Input: part model. Units: mm. Frame: model coordinates. A direction names the side the tool comes from. Give positions to 0.01 mm unless a question says otherwise; leave off trailing zeros. Order: outer loops, then holes, each group sorted by start corner. A loop starts at its lowest first (then second) coordinate and runs counter-clockwise, first axis right, second up.
```python
from build123d import *

# Parameters (mm, degrees)
SKETCH1_W           = 52
SKETCH1_H           = 40.7
SKETCH1_R           = 1.8
BOSS_EXTRUDE1_DEPTH = 1.6
SKETCH2_W           = 11
SKETCH2_H           = 10.7
SKETCH2_H_2         = 10
SKETCH2_H_3         = 13
BOSS_EXTRUDE2_DEPTH = 10
SKETCH3_R           = 1
CUT_EXTRUDE1_DEPTH  = 67.786899913


with BuildPart() as part:
    # Sketch1 → Boss-Extrude1 (new body)
    with BuildSketch(Plane(origin=(0, 0, 0), x_dir=(1, 0, 0), z_dir=(0, 1, 0))):
        with Locations((26, 20.35)):
            Rectangle(SKETCH1_W, SKETCH1_H)
        with Locations(Location((3.8, 36.85, 0), (0, 0, 270))):
            Circle(SKETCH1_R, mode=Mode.SUBTRACT)
        with Locations(Location((48.2, 36.85, 0), (0, 0, 270))):
            Circle(SKETCH1_R, mode=Mode.SUBTRACT)
        with Locations(Location((48.2, 3.85, 0), (0, 0, 270))):
            Circle(SKETCH1_R, mode=Mode.SUBTRACT)
        with Locations(Location((3.8, 3.85, 0), (0, 0, 270))):
            Circle(SKETCH1_R, mode=Mode.SUBTRACT)
    extrude(amount=BOSS_EXTRUDE1_DEPTH)

    # Sketch2 → Boss-Extrude2 (add)
    with BuildSketch(Plane(origin=(0, 1.6, 0), x_dir=(1, 0, 0), z_dir=(0, 1, 0))):
        with Locations((46.5, 15.35)):
            Rectangle(SKETCH2_W, SKETCH2_H)
        with Locations((5.5, 27.7)):
            Rectangle(SKETCH2_W, SKETCH2_H_2)
        with Locations((5.5, 14.2)):
            Rectangle(SKETCH2_W, SKETCH2_H_3)
    extrude(amount=BOSS_EXTRUDE2_DEPTH)

    # Sketch3 → Cut-Extrude1 (cut, through all)
    with BuildSketch(Plane(origin=(0, 1.6, 0), x_dir=(1, 0, 0), z_dir=(0, 1, 0))):
        with Locations(Location((46, 25.7, 0), (0, 0, 270))):
            Circle(SKETCH3_R)
        with Locations(Location((43, 25.7, 0), (0, 0, 270))):
            Circle(SKETCH3_R)
        with Locations(Location((40, 25.7, 0), (0, 0, 270))):
            Circle(SKETCH3_R)
        with Locations(Location((43, 28.7, 0), (0, 0, 270))):
            Circle(SKETCH3_R)
        with Locations(Location((40, 28.7, 0), (0, 0, 270))):
            Circle(SKETCH3_R)
        with Locations(Location((46, 28.7, 0), (0, 0, 270))):
            Circle(SKETCH3_R)
    extrude(amount=-CUT_EXTRUDE1_DEPTH, mode=Mode.SUBTRACT)


solid = part.part
```
1) Pull-direction query (X, two-part tool) for faces 1 (the face through (5, 7, -22.7)), 2 (the face through (11, 7, -28)), 3 (the face through (2.043, 0.789, -4.24)); classes: pulls with the +X half, pulls with the -X half, needs draft (parallel to the pull), parting line crosses it, or undercut.
2) Cut plane D-D (z = -18). Return the cut outline in (x, y).
3) Cut plane C-C (y = 3.75). Return the cut outline in (x, z).
4) Line query: probe 1 along X at (y, z) = (0.95, -36.85); probe 2 along X at (y, z) = (0.45, -28.7); probe 3 along X at (y, z) = (6, -16). Output: solid intervals per line, ascending.
5) Cut plane B-B (x = 48.2). Return the cut outline in (y, z).
6) Reachability of faces 4 (the face through (46, 7, -10)), 5 (the face through (46, 7, -20.7)), 6 (the face through (5, 7, -20.7)), 7 (the face through (26, 1, 0)), 8 (the face through (26, 1, -40.7)) from +Z, -Z, +X, -X, +Y, -Y: full face, straight path, thin tool, end or side. Return the list, or none.
7) Cut plane A-A (z = -28.7). Return the cut outline in (x, y), then the cut area to 3 significant figures.
8) First-contact query: P1, Ø1.5, axis at x = 17.5, z = -23, coming from the +Y side; P2, Ø3, axis at y = 7, z = -25, coming from the +X side; P3, Ø6, axis at x = 35, y = 2.5, coming from the -Z side; P4, Ø3, axis at x = 4.5, y = 6, coming from the +Z side. Flat tips, straight axial feed; report the tip coordinate or a pass-through.
Geometry says:
1. face 1: needs draft
1. face 2: pulls with the +X half
1. face 3: undercut
2. outline: (0, 0) - (52, 0) - (52, 11.6) - (41, 11.6) - (41, 1.6) - (11, 1.6) - (11, 11.6) - (0, 11.6) - close
3. outline: (0, -32.7) - (11, -32.7) - (11, -22.7) - (0, -22.7) - close; (0, -20.7) - (11, -20.7) - (11, -7.7) - (0, -7.7) - close; (41, -20.7) - (52, -20.7) - (52, -10) - (41, -10) - close
4. probe 1: x = 0 to 2, 5.6 to 46.4, 50 to 52
4. probe 2: x = 0 to 39, 41 to 42, 44 to 45, 47 to 52
4. probe 3: x = 0 to 11, 41 to 52
5. outline: (0, -40.7) - (1.6, -40.7) - (1.6, -38.65) - (0, -38.65) - close; (0, -35.05) - (1.6, -35.05) - (1.6, -20.7) - (11.6, -20.7) - (11.6, -10) - (1.6, -10) - (1.6, -5.65) - (0, -5.65) - close; (0, -2.05) - (1.6, -2.05) - (1.6, 0) - (0, 0) - close
6. face 4: +Z, +X, +Y
6. face 5: -Z, +X, -X, +Y
6. face 6: +X, -X, +Y
6. face 7: +Z, +X, -X, +Y, -Y
6. face 8: -Z, +X, -X, +Y, -Y
7. outline: (0, 0) - (39, 0) - (39, 1.6) - (11, 1.6) - (11, 11.6) - (0, 11.6) - close; (41, 0) - (42, 0) - (42, 1.6) - (41, 1.6) - close; (44, 0) - (45, 0) - (45, 1.6) - (44, 1.6) - close; (47, 0) - (52, 0) - (52, 1.6) - (47, 1.6) - close
7. area: 184 mm2
8. P1: stops at y = 1.6
8. P2: stops at x = 11
8. P3: stops at z = -40.7
8. P4: stops at z = -7.7
